CAD build for the part. Positions are in the model's coordinates, mm. Face numbers are marked on the shaded views. Give positions to 0.01 mm unless a question says otherwise; leave off trailing zeros. Loops run counter-clockwise (first coordinate to the right, second up) from the corner with the lowest first, then second, coordinate; pieces in that order, holes last. Notation, with made-up numbers: M 16.5,65.25 L 25.5,65.25 A16 cw 25.5,89.25 Z; hole C 83.5,58 d11. An arc over 180 degrees is marked long. Answer as CSV lines item,"result".
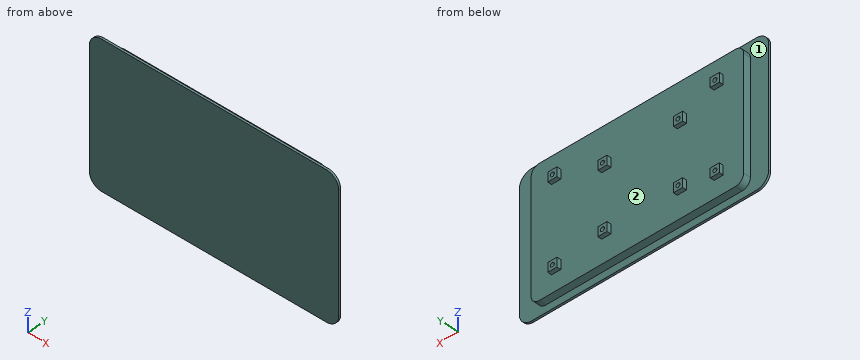
from build123d import *

# Parameters (mm, degrees)
BOSS_EXTRUDE1_DEPTH = 1.5875
BOSS_EXTRUDE2_DEPTH = 5.55625
SKETCH3_W           = 7.14375
SKETCH3_H           = 7.14375
SKETCH3_R           = 1.5875
BOSS_EXTRUDE3_DEPTH = 3.175
SKETCH4_W           = 7.14502
SKETCH4_H           = 7.14502
SKETCH4_R           = 1.5875
BOSS_EXTRUDE4_DEPTH = 3.175


with BuildPart() as part:
    # Sketch1 → Boss-Extrude1 (new body)
    with BuildSketch(Plane(origin=(0, 0, 0), x_dir=(1, 0, 0), z_dir=(0, 1, 0))):
        with BuildLine():
            Line((87.3125, 55.5625), (-87.3125, 55.5625))
            ThreePointArc((-87.3125, 55.5625), (-94.047692091, 52.772692091), (-96.8375, 46.0375))
            Line((-96.8375, 46.0375), (-96.8375, -46.0375))
            ThreePointArc((-96.8375, -46.0375), (-94.047692091, -52.772692091), (-87.3125, -55.5625))
            Line((-87.3125, -55.5625), (87.3125, -55.5625))
            ThreePointArc((87.3125, -55.5625), (94.047692091, -52.772692091), (96.8375, -46.0375))
            Line((96.8375, -46.0375), (96.8375, 46.0375))
            ThreePointArc((96.8375, 46.0375), (94.047692091, 52.772692091), (87.3125, 55.5625))
        make_face()
    extrude(amount=BOSS_EXTRUDE1_DEPTH)

    # Sketch2 → Boss-Extrude2 (add)
    with BuildSketch(Plane(origin=(0, 1.5875, 0), x_dir=(1, 0, 0), z_dir=(0, 1, 0))):
        with BuildLine():
            Line((76.2, 50.00625), (-76.2, 50.00625))
            ThreePointArc((-76.2, 50.00625), (-80.690128061, 48.146378061), (-82.55, 43.65625))
            Line((-82.55, 43.65625), (-82.55, -43.65625))
            ThreePointArc((-82.55, -43.65625), (-80.690128061, -48.146378061), (-76.2, -50.00625))
            Line((-76.2, -50.00625), (76.2, -50.00625))
            ThreePointArc((76.2, -50.00625), (80.690128061, -48.146378061), (82.55, -43.65625))
            Line((82.55, -43.65625), (82.55, 43.65625))
            ThreePointArc((82.55, 43.65625), (80.690128061, 48.146378061), (76.2, 50.00625))
        make_face()
    extrude(amount=BOSS_EXTRUDE2_DEPTH)

    # Sketch3 → Boss-Extrude3 (add)
    # profile 1 of 4: a face of its own
    with BuildSketch(Plane(origin=(0, 7.14375, 0), x_dir=(1, 0, 0), z_dir=(0, 1, 0))):
        with Locations((-63.103125, -32.940625)):
            Rectangle(SKETCH3_W, SKETCH3_H)
        with Locations(Location((-63.103125, -32.940625, 0), (0, 0, 270))):
            Circle(SKETCH3_R, mode=Mode.SUBTRACT)
    # profile 2 of 4: a face of its own
    with BuildSketch(Plane(origin=(0, 7.14375, 0), x_dir=(1, 0, 0), z_dir=(0, 1, 0))):
        with Locations((63.103125, -32.940625)):
            Rectangle(SKETCH3_W, SKETCH3_H)
        with Locations(Location((63.103125, -32.940625, 0), (0, 0, 90))):
            Circle(SKETCH3_R, mode=Mode.SUBTRACT)
    # profile 3 of 4: a face of its own
    with BuildSketch(Plane(origin=(0, 7.14375, 0), x_dir=(1, 0, 0), z_dir=(0, 1, 0))):
        with Locations((63.103125, 32.940625)):
            Rectangle(SKETCH3_W, SKETCH3_H)
        with Locations(Location((63.103125, 32.940625, 0), (0, 0, 270))):
            Circle(SKETCH3_R, mode=Mode.SUBTRACT)
    # profile 4 of 4: a face of its own
    with BuildSketch(Plane(origin=(0, 7.14375, 0), x_dir=(1, 0, 0), z_dir=(0, 1, 0))):
        with Locations((-63.103125, 32.940625)):
            Rectangle(SKETCH3_W, SKETCH3_H)
        with Locations(Location((-63.103125, 32.940625, 0), (0, 0, 90))):
            Circle(SKETCH3_R, mode=Mode.SUBTRACT)
    extrude(amount=BOSS_EXTRUDE3_DEPTH)

    # Sketch4 → Boss-Extrude4 (add)
    # profile 1 of 4: a face of its own
    with BuildSketch(Plane(origin=(0, 7.14375, 0), x_dir=(1, 0, 0), z_dir=(0, 1, 0))):
        with Locations((24.20874, -20.23999)):
            Rectangle(SKETCH4_W, SKETCH4_H)
        with Locations(Location((24.20874, -20.23999, 0), (0, 0, 270))):
            Circle(SKETCH4_R, mode=Mode.SUBTRACT)
    # profile 2 of 4: a face of its own
    with BuildSketch(Plane(origin=(0, 7.14375, 0), x_dir=(1, 0, 0), z_dir=(0, 1, 0))):
        with Locations((-34.52749, -20.23999)):
            Rectangle(SKETCH4_W, SKETCH4_H)
        with Locations(Location((-34.52749, -20.23999, 0), (0, 0, 90))):
            Circle(SKETCH4_R, mode=Mode.SUBTRACT)
    # profile 3 of 4: a face of its own
    with BuildSketch(Plane(origin=(0, 7.14375, 0), x_dir=(1, 0, 0), z_dir=(0, 1, 0))):
        with Locations((-34.52749, 28.17749)):
            Rectangle(SKETCH4_W, SKETCH4_H)
        with Locations(Location((-34.52749, 28.17749, 0), (0, 0, 270))):
            Circle(SKETCH4_R, mode=Mode.SUBTRACT)
    # profile 4 of 4: a face of its own
    with BuildSketch(Plane(origin=(0, 7.14375, 0), x_dir=(1, 0, 0), z_dir=(0, 1, 0))):
        with Locations((24.20874, 28.17749)):
            Rectangle(SKETCH4_W, SKETCH4_H)
        with Locations(Location((24.20874, 28.17749, 0), (0, 0, 90))):
            Circle(SKETCH4_R, mode=Mode.SUBTRACT)
    extrude(amount=BOSS_EXTRUDE4_DEPTH)


solid = part.part
1) Band-saw the part on B-B on z = 26. Give the cut face in (x, y), and give its area (3 significant figures).
Answer below:
outline,"M -96.84,0 L 96.84,0 L 96.84,1.59 L 82.55,1.59 L 82.55,7.14 L -82.55,7.14 L -82.55,1.59 L -96.84,1.59 Z"
area,"1,220 mm^2"
2) Drill centre lines: line 1 (X direction, y = 8, z = -35) (3 decimals); line 2 (Z direction, x = -63.5, y = 7.25); line 3 (X direction, y = 7.25, z = -34) (3 decimals). Where is each one in solid material? Low to high. Write a range as from..to.
Answer below:
line 1,"x = -66.675..-59.531, 59.531..66.675"
line 2,"z = -36.51..-34.48, -31.4..-29.37, 29.37..31.4, 34.48..36.51"
line 3,"x = -66.675..-64.285, -61.921..-59.531, 59.531..61.921, 64.285..66.675"
3) Mould opens along X. For the marked faces 1 and 2 say: +X half, -X half, draft (parallel to the pull), parting line (faces both ways), or undercut.
Answer below:
face 1,"draft"
face 2,"undercut"
4) Flat gauge pins, fed straight in: pin 1 (1.6 mm diameter, centred on x = 62.5, z = -32.5, fed in from +Y); pin 2 (3.5 mm diameter, centred on y = 9, z = 19, fed in from +X); pin 3 (5 mm diameter, centred on x = -37, y = 8, fed in from +Z). Where does each tip first touch, or does it go through?
Answer below:
pin 1,"stops at y = 7.14"
pin 2,"stops at x = 27.78"
pin 3,"stops at z = 50.01"
5) Band-saw the part on A-A on x = 7. Give the cut face in (y, z), and give its area (3 significant figures).
Answer below:
outline,"M 0,-55.56 L 1.59,-55.56 L 1.59,-50.01 L 7.14,-50.01 L 7.14,50.01 L 1.59,50.01 L 1.59,55.56 L 0,55.56 Z"
area,"732 mm^2"
